```python
from build123d import *

# Parameters (mm, degrees)
SKETCH_1_R               = 9
SKETCH_1_R_2             = 6.25
EXTRUDE_1_DEPTH          = 190
SKETCH_2_R               = 1.75
CUT_EXTRUDE_1_DEPTH      = 10
CUT_EXTRUDE_1_DEPTH_BACK = 10


with BuildPart() as part:
    # ｽｹｯﾁ1 → ﾎﾞｽ - 押し出し1 (new body)
    with BuildSketch(Plane.XY):
        Circle(SKETCH_1_R)
        Circle(SKETCH_1_R_2, mode=Mode.SUBTRACT)
    extrude(amount=EXTRUDE_1_DEPTH)

    # ｽｹｯﾁ2 → ｶｯﾄ - 押し出し1 (cut, two sides)
    with BuildSketch(Plane(origin=(0, 0, 0), x_dir=(0, 0, -1), z_dir=(1, 0, 0))) as cut_extrude_1_sk:
        with Locations((-7.5, 0)):
            Circle(SKETCH_2_R)
        with Locations((-182.5, 0)):
            Circle(SKETCH_2_R)
        with Locations((-45, 0)):
            Circle(SKETCH_2_R)
    extrude(amount=CUT_EXTRUDE_1_DEPTH, mode=Mode.SUBTRACT)
    extrude(cut_extrude_1_sk.sketch, amount=-CUT_EXTRUDE_1_DEPTH_BACK, mode=Mode.SUBTRACT)


solid = part.part
```
Could you check a few things on this model? Use its own coordinates, in mm. Give positions to 0.01 mm unless a question says otherwise; leave off trailing zeros. Loops run counter-clockwise (first coordinate to the right, second up) from the corner with the lowest first, then second, coordinate; pieces in that order, holes last. Notation, with made-up numbers: (-35, 11.5) - (22, 11.5) arc R23 cw to (22, 32.5) - close; hole circle Ø3 at (47.5, -35.75). An arc over 180 degrees is marked (long way). Answer in a Markdown table with one row per item. Add a question column.
Q1. We'd pull the mould along X, two halves only. Please class faces 1 (the face through (-1.172, 8.923, 93.67)), 2 (the face through (-7.479, 1.735, 45.228)), 3 (the face through (5.96, 1.88, 93.67)): +X half, -X half, draft (parallel to the pull), parting line (faces both ways), or undercut.
Q2. For pin 1 (3 mm diameter, centred on x = -6, z = 31.5, fed in from -Y); pin 2 (5 mm diameter, centred on x = -5, z = 64, fed in from -Y), each with a flat end and sliding along its axis, tell me the tip position at first contact or that it passes through.
Q3. If we section it at B-B (y = 0): State how many separate pieces and enclosed holes the cut face has, plus the area to 3 significant figures.
Q4. If we section it at A-A (x = 0): List the corners of the cut face in (y, z) for me.
Q5. If we section it at D-D (z = 34.5): List the corners of the cut face in (x, y) for me.
Q6. If we section it at C-C (z = 182.5): List the corners of the cut face in (x, y) for me, plus the area to 3 significant figures.
Q7. Please list where these lines run through material, in increasing order: L1, parallel to Z at x = 7.15, y = 0; L2, parallel to X at y = 0, z = 78; L3, parallel to Z at x = -7.75, y = 0.75. Write a range as from..to.
The answers:
| question | item | result |
|---|---|---|
| 1 | face 1 | parting line |
| 1 | face 2 | draft |
| 1 | face 3 | undercut |
| 2 | pin 1 | stops at y = -7.79 |
| 2 | pin 2 | stops at y = -8.65 |
| 3 | separate pieces | 8 |
| 3 | enclosed holes | 0 |
| 3 | area | 987 mm^2 |
| 4 | outline | (-9, 0) - (-6.25, 0) - (-6.25, 190) - (-9, 190) - close; (6.25, 0) - (9, 0) - (9, 190) - (6.25, 190) - close |
| 5 | outline | circle Ø18 at (0, 0); hole circle Ø12.5 at (0, 0) |
| 6 | outline | (-8.83, -1.75) arc R9 ccw to (8.83, -1.75) - (6, -1.75) arc R6.25 cw to (-6, -1.75) - close; (-8.83, 1.75) - (-6, 1.75) arc R6.25 cw to (6, 1.75) - (8.83, 1.75) arc R9 ccw to start |
| 6 | area | 112 mm^2 |
| 7 | L1 | z = 0..5.75, 9.25..43.25, 46.75..180.75, 184.25..190 |
| 7 | L2 | x = -9..-6.25, 6.25..9 |
| 7 | L3 | z = 0..5.92, 9.08..43.42, 46.58..180.92, 184.08..190 |
